```python
from build123d import *

# Parameters (mm, degrees)
SKETCH1_W           = 76.2
SKETCH1_H           = 127
BOSS_EXTRUDE1_DEPTH = 12.7
CUT_EXTRUDE1_DEPTH  = 6.35
CUT_EXTRUDE2_DEPTH  = 6.35
SKETCH4_W           = 9.525
SKETCH4_H           = 12.7
CUT_EXTRUDE3_DEPTH  = 2.2225
SKETCH5_R           = 2.0828
CUT_EXTRUDE4_DEPTH  = 25.4


with BuildPart() as part:
    # Sketch1 → Boss-Extrude1 (new body)
    with BuildSketch(Plane.XY):
        with Locations((38.1, 63.5)):
            Rectangle(SKETCH1_W, SKETCH1_H)
    extrude(amount=BOSS_EXTRUDE1_DEPTH)

    # Sketch2 → Cut-Extrude1 (cut)
    with BuildSketch(Plane.XY.offset(12.7)):
        with BuildLine():
            Line((71.4375, 12.7), (71.4375, 25.4))
            ThreePointArc((71.4375, 25.4), (69.85, 26.9875), (68.2625, 25.4))
            Line((68.2625, 25.4), (68.2625, 12.7))
            ThreePointArc((68.2625, 12.7), (69.85, 11.1125), (71.4375, 12.7))
        make_face()
        with BuildLine():
            Line((7.9375, 12.7), (7.9375, 25.4))
            ThreePointArc((7.9375, 25.4), (6.35, 26.9875), (4.7625, 25.4))
            Line((4.7625, 25.4), (4.7625, 12.7))
            ThreePointArc((4.7625, 12.7), (6.35, 11.1125), (7.9375, 12.7))
        make_face()
        with BuildLine():
            Line((7.9375, 101.6), (7.9375, 114.3))
            ThreePointArc((7.9375, 114.3), (6.35, 115.8875), (4.7625, 114.3))
            Line((4.7625, 114.3), (4.7625, 101.6))
            ThreePointArc((4.7625, 101.6), (6.35, 100.0125), (7.9375, 101.6))
        make_face()
        with BuildLine():
            Line((71.4375, 101.6), (71.4375, 114.3))
            ThreePointArc((71.4375, 114.3), (69.85, 115.8875), (68.2625, 114.3))
            Line((68.2625, 114.3), (68.2625, 101.6))
            ThreePointArc((68.2625, 101.6), (69.85, 100.0125), (71.4375, 101.6))
        make_face()
    extrude(amount=-CUT_EXTRUDE1_DEPTH, mode=Mode.SUBTRACT)

    # Sketch3 → Cut-Extrude2 (cut)
    with BuildSketch(Plane(origin=(0, 0, 0), x_dir=(-1, 0, 0), z_dir=(0, 0, -1))):
        with BuildLine():
            Line((-23.6855, 96.8375), (-10.9855, 96.8375))
            ThreePointArc((-10.9855, 96.8375), (-9.398, 98.425), (-10.9855, 100.0125))
            Line((-10.9855, 100.0125), (-23.6855, 100.0125))
            ThreePointArc((-23.6855, 100.0125), (-25.273, 98.425), (-23.6855, 96.8375))
        make_face()
        with BuildLine():
            Line((-65.0875, 96.8375), (-52.3875, 96.8375))
            ThreePointArc((-52.3875, 96.8375), (-50.8, 98.425), (-52.3875, 100.0125))
            Line((-52.3875, 100.0125), (-65.0875, 100.0125))
            ThreePointArc((-65.0875, 100.0125), (-66.675, 98.425), (-65.0875, 96.8375))
        make_face()
        with BuildLine():
            Line((-65.0875, 26.9875), (-52.3875, 26.9875))
            ThreePointArc((-52.3875, 26.9875), (-50.8, 28.575), (-52.3875, 30.1625))
            Line((-52.3875, 30.1625), (-65.0875, 30.1625))
            ThreePointArc((-65.0875, 30.1625), (-66.675, 28.575), (-65.0875, 26.9875))
        make_face()
        with BuildLine():
            Line((-23.6855, 26.9875), (-10.9855, 26.9875))
            ThreePointArc((-10.9855, 26.9875), (-9.398, 28.575), (-10.9855, 30.1625))
            Line((-10.9855, 30.1625), (-23.6855, 30.1625))
            ThreePointArc((-23.6855, 30.1625), (-25.273, 28.575), (-23.6855, 26.9875))
        make_face()
    extrude(amount=-CUT_EXTRUDE2_DEPTH, mode=Mode.SUBTRACT)

    # Sketch4 → Cut-Extrude3 (cut)
    with BuildSketch(Plane.XY.offset(12.7)):
        with Locations((38.1, 50.8)):
            Rectangle(SKETCH4_W, SKETCH4_H)
    extrude(amount=-CUT_EXTRUDE3_DEPTH, mode=Mode.SUBTRACT)

    # Sketch5 → Cut-Extrude4 (cut)
    with BuildSketch(Plane.XY.offset(12.7)):
        with Locations((12.7, 82.55)):
            Circle(SKETCH5_R)
        with Locations((63.5, 82.55)):
            Circle(SKETCH5_R)
    extrude(amount=-CUT_EXTRUDE4_DEPTH, mode=Mode.SUBTRACT)


solid = part.part
```
Here's how the part is built. I have some questions about the finished solid (model axes, mm). A direction names the side the tool comes from. Coordinates: 2 decimals unless noted, no trailing zeros. Order: outer loops, then holes, each group sorted by start corner. A loop starts at its lowest first (then second) coordinate and runs counter-clockwise, first axis right, second up. Notation, with made-up numbers: M 29,65.25 L 64,65.25 A14 ccw 64,90.25 Z; hole C 82,65.25 d5. An arc over 180 degrees is marked long. Answer as a JSON object with one key per item and string values. Group by question number.
(1) For pin 1 (1 mm diameter, centred on x = 70, y = 22.5, fed in from +Z); pin 2 (5 mm diameter, centred on x = 40, y = 50.5, fed in from +Z), each with a flat end and sliding along its axis, tell me the tip position at first contact or that it passes through.
(2) I need wall thicknesses on probe 1 along Y at (x, z) = (63.5, 6); probe 2 along X at (y, z) = (46.5, 11.5); probe 3 along Y at (x, z) = (63.5, 10.25). Which ranges of each line are inside material? Lowest first, please.
(3) Suppose I cut it at A-A, the plane x = 63.5. Please give me the cut outline in (y, z).
(4) Suppose I cut it at D-D, the plane z = 2. State how many separate pieces and enclosed holes the cut face has, then the cut area to 3 significant figures.
(5) Suppose I cut it at B-B, the plane y = 82.55. Please give me the cut outline in (x, z).
(6) Which directions (+Z, -Z, +X, -X, +Y, -Y) give clear straight access to the entire face, cutting with the end or side of a thin tool? Please do faces 4 (the face through (12.429, 84.615, 6.439)), 5 (the face through (71.438, 19, 10)), 6 (the face through (17, 30.162, 3)).
(7) If we mould it in two halves opening along X, with no side actions, what happens to faces 1 (the face through (71.438, 108, 10)), 2 (the face through (76.2, 63, 6)), 3 (the face through (0, 63, 6))? For each: released by +X, released by -X, zero draft, split by the parting line, or undercut.
(8) Suppose I cut it at C-C, the plane x = 35.5. Please give me the cut outline in (y, z), then the cut area to 3 significant figures.
Values found:
{
 "1": {"pin 1": "stops at z = 6.35", "pin 2": "stops at z = 10.48"},
 "2": {"probe 1": "y = 0 to 26.99, 30.16 to 80.47, 84.63 to 96.84, 100.01 to 127", "probe 2": "x = 0 to 33.34, 42.86 to 76.2", "probe 3": "y = 0 to 80.47, 84.63 to 127"},
 "3": {"outline": "M 0,0 L 26.99,0 L 26.99,6.35 L 30.16,6.35 L 30.16,0 L 80.47,0 L 80.47,12.7 L 0,12.7 Z; M 84.63,0 L 96.84,0 L 96.84,6.35 L 100.01,6.35 L 100.01,0 L 127,0 L 127,12.7 L 84.63,12.7 Z"},
 "4": {"separate pieces": "1", "enclosed holes": "6", "area": "9,460 mm^2"},
 "5": {"outline": "M 0,0 L 10.62,0 L 10.62,12.7 L 0,12.7 Z; M 14.78,0 L 61.42,0 L 61.42,12.7 L 14.78,12.7 Z; M 65.58,0 L 76.2,0 L 76.2,12.7 L 65.58,12.7 Z"},
 "6": {"face 4": "+Z, -Z", "face 5": "+Z", "face 6": "-Z"},
 "7": {"face 1": "undercut", "face 2": "released by +X", "face 3": "released by -X"},
 "8": {"outline": "M 0,0 L 127,0 L 127,12.7 L 57.15,12.7 L 57.15,10.48 L 44.45,10.48 L 44.45,12.7 L 0,12.7 Z", "area": "1,580 mm^2"}
}
